from build123d import *

# Parameters (mm, degrees)
SKETCH1_W           = 27
SKETCH1_H           = 27
BOSS_EXTRUDE1_DEPTH = 27
CUT_EXTRUDE1_REACH  = 43.32
SKETCH2_W           = 25
SKETCH2_H           = 25
CUT_EXTRUDE2_REACH  = 45.313
SKETCH3_R           = 1.75
SKETCH3_R_2         = 1
SKETCH4_W           = 27
SKETCH4_H           = 68
BOSS_EXTRUDE2_DEPTH = 2
CUT_EXTRUDE3_REACH  = 92.375
SKETCH5_R           = 1.3
FILLET1_R           = 10


with BuildPart() as part:
    # Sketch1 → Boss-Extrude1 (new body)
    with BuildSketch(Plane(origin=(0, 0, 0), x_dir=(0, 1, 0), z_dir=(0, 0, 1))):
        with Locations((2.289473684, -9.347039474)):
            Rectangle(SKETCH1_W, SKETCH1_H)
    extrude(amount=BOSS_EXTRUDE1_DEPTH)

    # Sketch2 → Cut-Extrude1 (cut, up to next)
    with BuildSketch(Plane.YZ.offset(22.847039474), mode=Mode.PRIVATE) as cut_extrude1_sk1:
        with Locations((3.289473684, 14.5)):
            Rectangle(SKETCH2_W, SKETCH2_H)
    cut_extrude1_tool1 = extrude(cut_extrude1_sk1.sketch, amount=-CUT_EXTRUDE1_REACH, mode=Mode.PRIVATE) & part.part
    add(cut_extrude1_tool1.solids().sort_by_distance((22.847039, 3.289474, 14.5))[0], mode=Mode.SUBTRACT)

    # Sketch3 → Cut-Extrude2 (cut, up to next)
    with BuildSketch(Plane(origin=(0, -9.210526316, 0), x_dir=(-1, 0, 0), z_dir=(0, 1, 0)), mode=Mode.PRIVATE) as cut_extrude2_sk1:
        with Locations(Location((-9.347039474, 14.5, 0), (0, 0, 90))):
            Circle(SKETCH3_R)
    cut_extrude2_tool1 = extrude(cut_extrude2_sk1.sketch, amount=-CUT_EXTRUDE2_REACH, mode=Mode.PRIVATE) & part.part
    # Sketch3 → Cut-Extrude2 (cut, up to next)
    with BuildSketch(Plane(origin=(0, -9.210526316, 0), x_dir=(-1, 0, 0), z_dir=(0, 1, 0)), mode=Mode.PRIVATE) as cut_extrude2_sk2:
        with Locations(Location((-9.347039474, 23, 0), (0, 0, 90))):
            Circle(SKETCH3_R_2)
    cut_extrude2_tool2 = extrude(cut_extrude2_sk2.sketch, amount=-CUT_EXTRUDE2_REACH, mode=Mode.PRIVATE) & part.part
    # Sketch3 → Cut-Extrude2 (cut, up to next)
    with BuildSketch(Plane(origin=(0, -9.210526316, 0), x_dir=(-1, 0, 0), z_dir=(0, 1, 0)), mode=Mode.PRIVATE) as cut_extrude2_sk3:
        with Locations((-9.347039474, 6)):
            Circle(SKETCH3_R_2)
    cut_extrude2_tool3 = extrude(cut_extrude2_sk3.sketch, amount=-CUT_EXTRUDE2_REACH, mode=Mode.PRIVATE) & part.part
    add(cut_extrude2_tool1.solids().sort_by_distance((9.347039, -9.210526, 14.5))[0], mode=Mode.SUBTRACT)
    add(cut_extrude2_tool2.solids().sort_by_distance((9.347039, -9.210526, 23))[0], mode=Mode.SUBTRACT)
    add(cut_extrude2_tool3.solids().sort_by_distance((9.347039, -9.210526, 6))[0], mode=Mode.SUBTRACT)

    # Sketch4 → Boss-Extrude2 (add)
    with BuildSketch(Plane.XY.offset(2)):
        with Locations((9.347039474, 49.789473684)):
            Rectangle(SKETCH4_W, SKETCH4_H)
    extrude(amount=-BOSS_EXTRUDE2_DEPTH)

    # Sketch5 → Cut-Extrude3 (cut, up to next)
    with BuildSketch(Plane.XY.offset(2), mode=Mode.PRIVATE) as cut_extrude3_sk1:
        with Locations((1.347039474, -6.210526316)):
            Circle(SKETCH5_R)
    cut_extrude3_tool1 = extrude(cut_extrude3_sk1.sketch, amount=-CUT_EXTRUDE3_REACH, mode=Mode.PRIVATE) & part.part
    # Sketch5 → Cut-Extrude3 (cut, up to next)
    with BuildSketch(Plane.XY.offset(2), mode=Mode.PRIVATE) as cut_extrude3_sk2:
        with Locations((1.347039474, 78.789473684)):
            Circle(SKETCH5_R)
    cut_extrude3_tool2 = extrude(cut_extrude3_sk2.sketch, amount=-CUT_EXTRUDE3_REACH, mode=Mode.PRIVATE) & part.part
    # Sketch5 → Cut-Extrude3 (cut, up to next)
    with BuildSketch(Plane.XY.offset(2), mode=Mode.PRIVATE) as cut_extrude3_sk3:
        with Locations((17.347039474, -6.210526316)):
            Circle(SKETCH5_R)
    cut_extrude3_tool3 = extrude(cut_extrude3_sk3.sketch, amount=-CUT_EXTRUDE3_REACH, mode=Mode.PRIVATE) & part.part
    # Sketch5 → Cut-Extrude3 (cut, up to next)
    with BuildSketch(Plane.XY.offset(2), mode=Mode.PRIVATE) as cut_extrude3_sk4:
        with Locations((17.347039474, 78.789473684)):
            Circle(SKETCH5_R)
    cut_extrude3_tool4 = extrude(cut_extrude3_sk4.sketch, amount=-CUT_EXTRUDE3_REACH, mode=Mode.PRIVATE) & part.part
    add(cut_extrude3_tool1.solids().sort_by_distance((1.347039, -6.210526, 2))[0], mode=Mode.SUBTRACT)
    add(cut_extrude3_tool2.solids().sort_by_distance((1.347039, 78.789474, 2))[0], mode=Mode.SUBTRACT)
    add(cut_extrude3_tool3.solids().sort_by_distance((17.347039, -6.210526, 2))[0], mode=Mode.SUBTRACT)
    add(cut_extrude3_tool4.solids().sort_by_distance((17.347039, 78.789474, 2))[0], mode=Mode.SUBTRACT)

    # Fillet1
    fillet1_edges = [part.edges().sort_by_distance(p)[0] for p in [
        (-4.152960526, -10.210526316, 27),
        (22.847039474, -10.210526316, 27),
    ]]
    fillet(fillet1_edges, radius=FILLET1_R)


solid = part.part
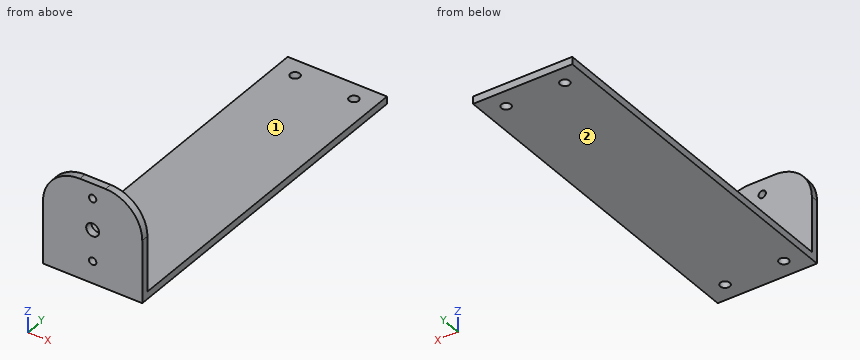
Design review of the part built by this model. Coordinates are the model's own, in mm. Face numbers are marked on the shaded views. A direction names the side the tool comes from. Give positions to 0.01 mm unless a question says otherwise; leave off trailing zeros. Write each loop counter-clockwise with the first axis right and the second up, starting at its lowest first coordinate (ties: lowest second). Pieces come first, ordered by that corner, then holes. Notation, with made-up numbers: M -32.5,46 L -12.5,46 A29 cw -12.5,84 Z; hole C -10,-30 d11. An arc over 180 degrees is marked long. Answer as a JSON object with one key per item and string values. Group by question number.
1) We need section A-A (z = 14.5). Give the boundary of the cut face in (x, y).
2) For line 1 along X through (y, z) = (-10.3, 14.5); line 2 along Z through (x, y) = (1, 46.5); line 3 along Y through (x, z) = (21, 17), list the stretches that pass through material, from the lowest coordinate up.
3) Clearance check with flat-ended pins moving along their axes: pin 1 Ø1.6 at (x, y) = (17.35, -6.21) entering from +Z; pin 2 Ø10 at (x, z) = (15, 22.5) entering from +Y; pin 3 Ø4 at (x, y) = (1.35, 78.79) entering from +Z. State where each tip first meets the part, or that it passes through.
4) We need section B-B (z = 6). Give the boundary of the cut face in (x, y), and give its area (3 significant figures).
5) We need section C-C (y = 70.5). Give the boundary of the cut face in (x, z).
6) Tool access review of the marked faces 1 and 2: name each direction out of +Z, -Z, +X, -X, +Y, -Y from which nothing blocks a thin tool from reaching the whole face with its end or side.
Answer key:
{
 "1": {"outline": "M -4.15,-11.21 L 7.6,-11.21 L 7.6,-9.21 L -4.15,-9.21 Z; M 11.1,-11.21 L 22.85,-11.21 L 22.85,-9.21 L 11.1,-9.21 Z"},
 "2": {"line 1": "x = -4.15 to 7.6, 11.1 to 22.85", "line 2": "z = 0 to 2", "line 3": "y = -11.21 to -9.21"},
 "3": {"pin 1": "passes through", "pin 2": "stops at y = -9.21", "pin 3": "stops at z = 2"},
 "4": {"outline": "M -4.15,-11.21 L 8.35,-11.21 L 8.35,-9.21 L -4.15,-9.21 Z; M 10.35,-11.21 L 22.85,-11.21 L 22.85,-9.21 L 10.35,-9.21 Z", "area": "50.0 mm²"},
 "5": {"outline": "M -4.15,0 L 22.85,0 L 22.85,2 L -4.15,2 Z"},
 "6": {"face 1": "+Z, +X, -X, +Y", "face 2": "-Z, +X, -X, +Y, -Y"}
}
